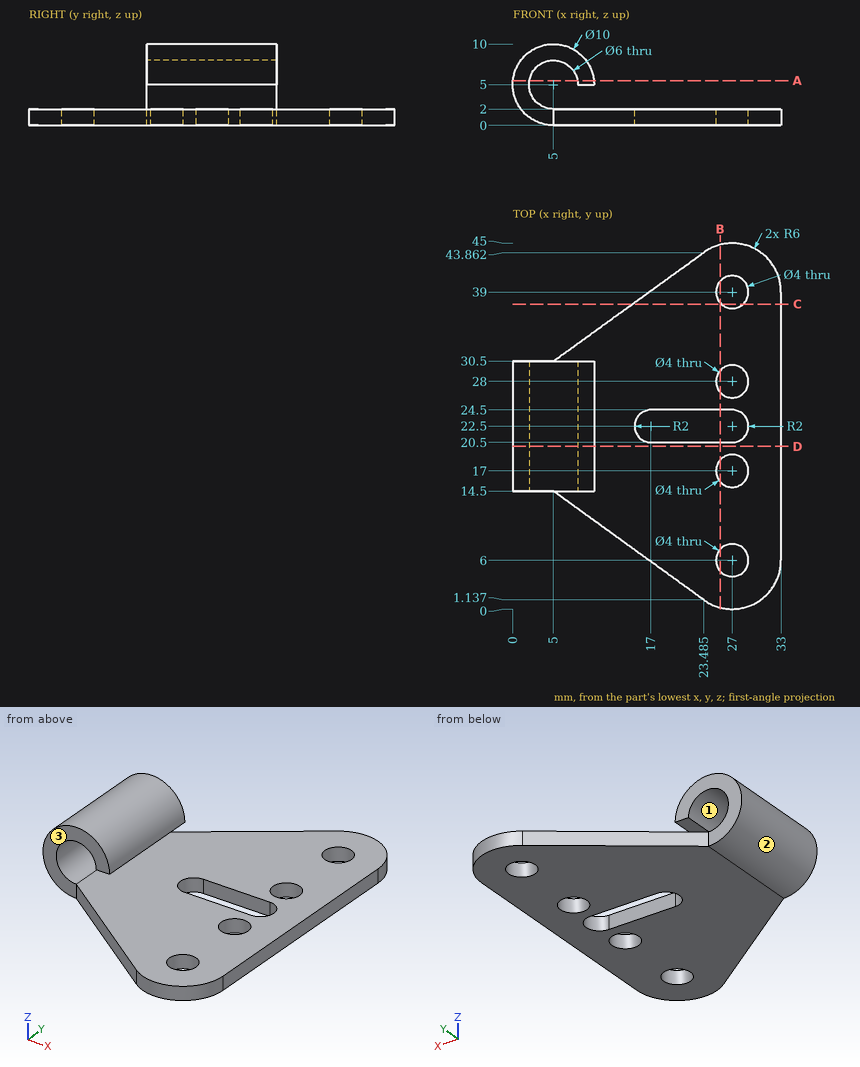
Geometry check sheet. Reference: drawing and pictorial views, mm from the part's lowest x, y, z. Coordinates: 2 decimals unless noted, no trailing zeros. Order: outer loops, then holes, each group sorted by start corner. A loop starts at its lowest first (then second) coordinate and runs counter-clockwise, first axis right, second up.
Item 1: Release check for a two-part mould opening along Z. For the marked faces 1, 2 and 3 record: +Z half, -Z half, draft (parallel to the pull), parting line (faces both ways), or undercut.
Filled in:
face 1: undercut
face 2: parting line
face 3: draft
Item 2: Depth check by flat-ended pin: pin 1 (1.6 mm diameter, centred on x = 23, z = 0.5, fed in from -Y) (1 decimal); pin 2 (8.5 mm diameter, centred on x = 21, y = 19, fed in from +Z); pin 3 (5 mm diameter, centred on y = 37, z = 3, fed in from -X); pin 4 (3 mm diameter, centred on x = 27, y = 39, fed in from +Z). Enter the tip coordinate at first touch or a pass-through.
Filled in:
pin 1: stops at y = 0.9
pin 2: stops at z = 2
pin 3: stops at x = 10.82
pin 4: passes through
Item 3: Material ranges on L1, parallel to Y at x = 27, z = 1.2; L2, parallel to Z at x = 31.5, y = 18.5; L3, parallel to Y at x = 8, z = 8, recorded low to high.
Filled in:
L1: y = 0 to 4, 8 to 15, 19 to 20.5, 24.5 to 26, 30 to 37, 41 to 45
L2: z = 0 to 2
L3: y = 14.5 to 30.5
Item 4: Section check D-D, the plane y = 20. Enter the section's corners in (x, z).
Filled in:
outline: (5, 0) - (33, 0) - (33, 2) - (5, 2) arc R3 cw (long way) to (8, 5) - (10, 5) arc R5 ccw (long way) to start
Item 5: Section check A-A, the plane z = 5.5. Enter the section's corners in (x, y) (1 decimal).
Filled in:
outline: (0, 14.5) - (2, 14.5) - (2, 30.5) - (0, 30.5) - close; (8, 14.5) - (10, 14.5) - (10, 30.5) - (8, 30.5) - close
Item 6: Section check C-C, the plane y = 37.5. Enter the section's corners in (x, z).
Filled in:
outline: (14.68, 0) - (25.68, 0) - (25.68, 2) - (14.68, 2) - close; (28.32, 0) - (33, 0) - (33, 2) - (28.32, 2) - close
Item 7: Section check B-B, the plane x = 25.5. Enter the section's corners in (y, z).
Filled in:
outline: (0.19, 0) - (4.68, 0) - (4.68, 2) - (0.19, 2) - close; (7.32, 0) - (15.68, 0) - (15.68, 2) - (7.32, 2) - close; (18.32, 0) - (20.5, 0) - (20.5, 2) - (18.32, 2) - close; (24.5, 0) - (26.68, 0) - (26.68, 2) - (24.5, 2) - close; (29.32, 0) - (37.68, 0) - (37.68, 2) - (29.32, 2) - close; (40.32, 0) - (44.81, 0) - (44.81, 2) - (40.32, 2) - close
